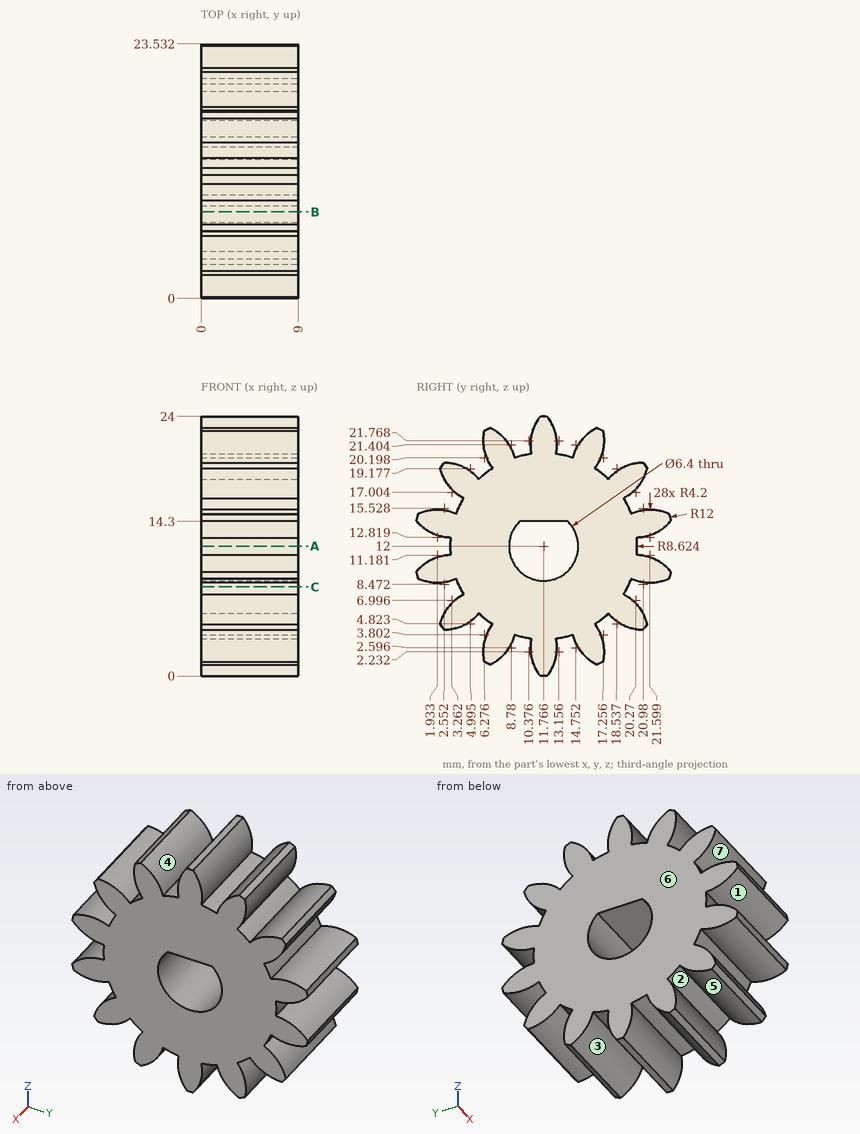
Design review of the part shown in the three views and the two pictorial views. Dimensions are in mm from the part's minimum x, y and z. A direction names the side the tool comes from. Round coordinates to 2 decimals unless told otherwise and drop trailing zeros. Loops run counter-clockwise (first coordinate to the right, second up) from the corner with the lowest first, then second, coordinate; pieces in that order, holes last.
(1) We need section A-A (z = 12). Give the boundary of the cut face in (x, y) (1 decimal).
Returned:
outline: (0, 3.1) - (9, 3.1) - (9, 8.6) - (0, 8.6) - close; (0, 15) - (9, 15) - (9, 20.4) - (0, 20.4) - close
(2) We need section C-C (z = 8.25). Give the boundary of the cut face in (x, y).
Returned:
outline: (0, 4) - (9, 4) - (9, 19.53) - (0, 19.53) - close
(3) Clearance check with flat-ended pins moving along their axes: P1, Ø1, axis at x = 1.5, z = 5.5, coming from the -Y side; P2, Ø4, axis at y = 11.77, z = 12, coming from the +X side. State where each tip first meets the part, or that it passes through.
Returned:
P1: stops at y = 2.25
P2: passes through
(4) Mouldability with a two-part tool opening along Z and no side actions: class the marked faces 5, 6 and 7 as released by +Z, released by -Z, zero draft, split by the parting line, or undercut.
Returned:
face 5: released by -Z
face 6: zero draft
face 7: undercut
(5) Tool access review of the marked faces 1, 2, 3 and 4: name each direction out of +Z, -Z, +X, -X, +Y, -Y from which nothing blocks a thin tool from reaching the whole face with its end or side.
Returned:
face 1: +X, -X, -Y
face 2: +X, -X
face 3: -Z, +X, -X
face 4: +Z, +X, -X
(6) We need section B-B (y = 8). Give the boundary of the cut face in (x, z), plus the area to 3 significant figures.
Returned:
outline: (0, 1.89) - (9, 1.89) - (9, 22.11) - (0, 22.11) - close
area: 182 mm2
(7) Wall thickness on line 1 along Y through (x, z) = (8.25, 22.5) (1 decimal); line 2 along Z through (x, y) = (3.5, 3.25) (1 decimal); line 3 along Y through (x, z) = (4, 3) (1 decimal): over which ranges is each line inside the solid? List them lowest first.
Returned:
line 1: y = 6.2 to 7.6, 10.7 to 12.8, 16 to 17.3
line 2: z = 4.3 to 6.7, 8.8 to 15.2, 17.3 to 19.7
line 3: y = 6.2 to 8.8, 10.6 to 13, 14.8 to 17.3
